Job drawing, mm, ordinate dimensions from the low corner. One solid piece. A direction names the side the tool comes from. Round coordinates to 2 decimals unless told otherwise and drop trailing zeros. Order: outer loops, then holes, each group sorted by start corner. A loop starts at its lowest first (then second) coordinate and runs counter-clockwise, first axis right, second up. Notation, with made-up numbers: (23, 84) -> (54, 84) arc R36 cw to (54, 118) -> close; hole circle Ø2 at (-15.5, -2.75). An arc over 180 degrees is marked (long way). Return JSON: item names as keys, results as strings. Group by question number.
Q1. Mould opens along Z. For the marked faces 1, 2, 3 and 4 say: +Z half, -Z half, draft (parallel to the pull), parting line (faces both ways), or undercut.
Q2. Which spindle directions (+Z, -Z, +X, -X, +Y, -Y) get a long thin tool onto all of the face, cutting with end or side? Do the marked faces 5, 6, 7, 8 and 9. Say none if no direction does.
Q3. Probe line 1 along X through (y, z) = (12, 53.5); line 2 along Z through (x, y) = (31, 6); line 3 along X through (y, z) = (31, 60.6). List the from-to ranges inside material, lowest first.
Q4. Cut at B-B (y = 31). Write the cut outline in (x, z), then the cut area to 3 significant figures.
Q5. Cut at D-D (y = 14). Count the separate pieces of the cut face and the enclosed holes in it, then the cut area to 3 significant figures.
Q6. Cut at A-A (x = 12). Write the cut outline in (y, z), then the cut area to 3 significant figures.
Q7. Flat gauge pins, fed straight in: pin 1 (1.5 mm diameter, centred on x = 38.5, z = 60, fed in from -Y); pin 2 (2 mm diameter, centred on x = 41.175, z = 53.475, fed in from +Y); pin 3 (14 mm diameter, centred on x = 27, z = 34, fed in from +Y); pin 4 (12 mm diameter, centred on y = 9.5, z = 16, fed in from +X). Where does each tip first touch, or does it go through?
Q8. Cut at C-C (x = 33.65). Write the cut outline in (y, z), then the cut area to 3 significant figures.
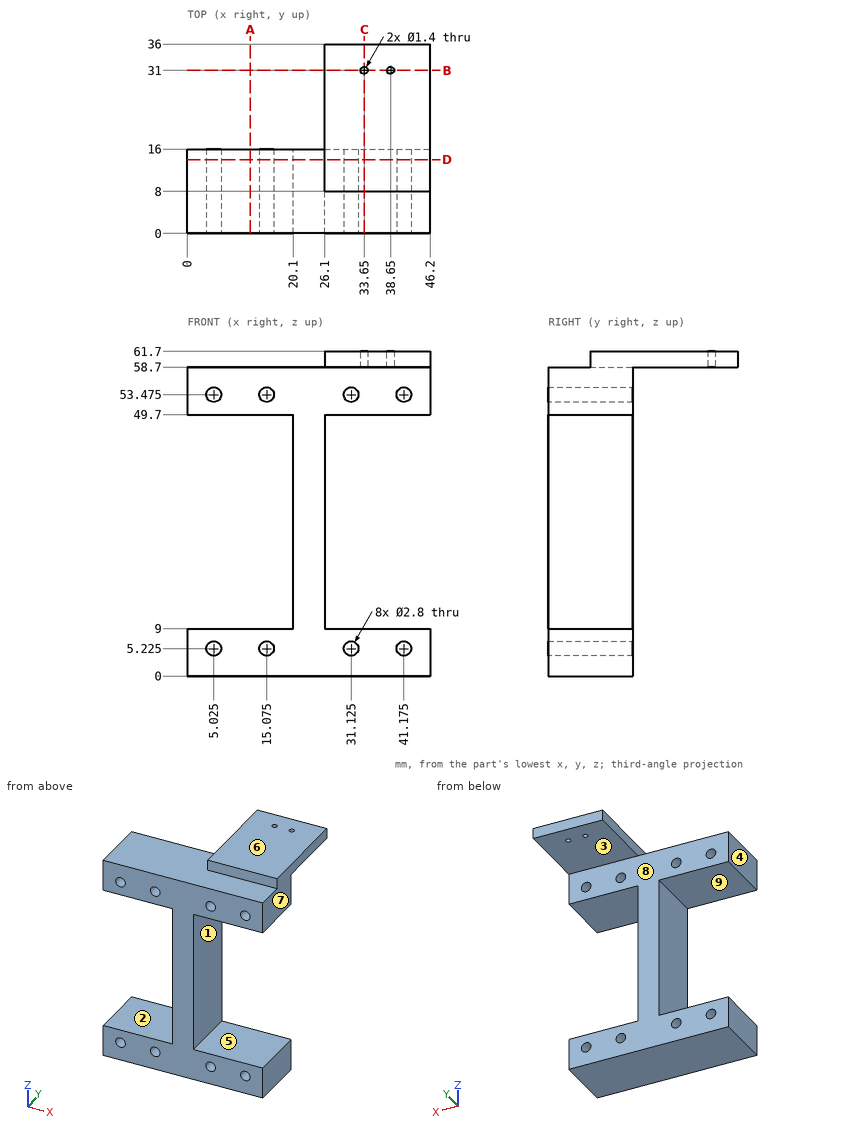
Solution:
{
 "1": {"face 1": "undercut", "face 2": "undercut", "face 3": "-Z half", "face 4": "draft"},
 "2": {"face 5": "+X, +Y, -Y", "face 6": "+Z, +X, -X, +Y, -Y", "face 7": "+Z, -Z, +X, +Y, -Y", "face 8": "-Z, +X, -X, +Y", "face 9": "-X, +Y, -Y"},
 "3": {"line 1": "x = 0 to 3.63, 6.42 to 13.68, 16.47 to 29.73, 32.52 to 39.78, 42.57 to 46.2", "line 2": "z = 0 to 3.83, 6.62 to 9, 49.7 to 52.08, 54.87 to 58.7", "line 3": "x = 26.1 to 32.95, 34.35 to 37.95, 39.35 to 46.2"},
 "4": {"outline": "(26.1, 58.7) -> (32.95, 58.7) -> (32.95, 61.7) -> (26.1, 61.7) -> close; (34.35, 58.7) -> (37.95, 58.7) -> (37.95, 61.7) -> (34.35, 61.7) -> close; (39.35, 58.7) -> (46.2, 58.7) -> (46.2, 61.7) -> (39.35, 61.7) -> close", "area": "51.9 mm²"},
 "5": {"separate pieces": "1", "enclosed holes": "8", "area": "1,090 mm²"},
 "6": {"outline": "(0, 0) -> (16, 0) -> (16, 9) -> (0, 9) -> close; (0, 49.7) -> (16, 49.7) -> (16, 58.7) -> (0, 58.7) -> close", "area": "288 mm²"},
 "7": {"pin 1": "stops at y = 8", "pin 2": "passes through", "pin 3": "stops at y = 16", "pin 4": "stops at x = 26.1"},
 "8": {"outline": "(0, 0) -> (16, 0) -> (16, 9) -> (0, 9) -> close; (0, 49.7) -> (16, 49.7) -> (16, 58.7) -> (30.3, 58.7) -> (30.3, 61.7) -> (8, 61.7) -> (8, 58.7) -> (0, 58.7) -> close; (31.7, 58.7) -> (36, 58.7) -> (36, 61.7) -> (31.7, 61.7) -> close", "area": "368 mm²"}
}
